```python
from build123d import *

# Parameters (mm, degrees)
F0_W     = 12.065
F0_H     = 4.572
F1_DEPTH = 17.272
F2_W     = 12.065
F2_H     = 2.794
F2_W_2   = 1.0795
F2_H_2   = 1.778
F3_DEPTH = 21.59


with BuildPart() as f1:
    # F0 (on Front) → F1 (new body)
    with BuildSketch(Plane.XZ):
        Rectangle(F0_W, F0_H)
    extrude(amount=F1_DEPTH)

    # F2 (on face) → F3 (join)
    with BuildSketch(Plane(origin=(0, 0, 0), x_dir=(-1, 0, 0), z_dir=(0, 1, 0))):
        with Locations((0, 0.889)):
            Rectangle(F2_W, F2_H)
        with Locations((6.57225, -1.397)):
            Rectangle(F2_W_2, F2_H_2)
        with Locations((0, -1.397)):
            Rectangle(F2_W, F2_H_2)
        with Locations((-6.57225, -1.397)):
            Rectangle(F2_W_2, F2_H_2)
    extrude(amount=F3_DEPTH)


solid = f1.part
```
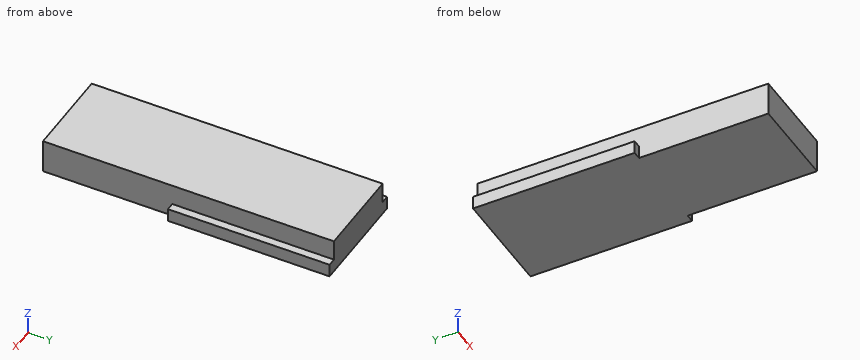
The model under review builds one solid part; all positions refer to its coordinate system, in mm. Round coordinates to 2 decimals unless told otherwise and drop trailing zeros. Order: outer loops, then holes, each group sorted by start corner. A loop starts at its lowest first (then second) coordinate and runs counter-clockwise, first axis right, second up. Notation, with made-up numbers: (77, 16) -> (103, 16) arc R27 cw to (103, 53) -> close; hole circle Ø11 at (0.5, 35). An arc over 180 degrees is marked (long way). Use a Markdown table: item, result.
Q1. Clearance check with flat-ended pins moving along their axes: P1, Ø1.5, axis at y = 0.5, z = 1.5, coming from the -X side; P2, Ø1.2, axis at x = 7, y = 8, coming from the +Z side. State where each tip first meets the part, or that it passes through.
Values:
| item | result |
|---|---|
| P1 | stops at x = -6.03 |
| P2 | stops at z = -0.51 |
Q2. We need section A-A on y = 12. Write out the cut boundary in (x, z).
Values:
| item | result |
|---|---|
| outline | (-7.11, -2.29) -> (7.11, -2.29) -> (7.11, -0.51) -> (6.03, -0.51) -> (6.03, 2.29) -> (-6.03, 2.29) -> (-6.03, -0.51) -> (-7.11, -0.51) -> close |
Q3. We need section C-C on z = 0.5. Write out the cut boundary in (x, y), then the cut area to 3 significant figures.
Values:
| item | result |
|---|---|
| outline | (-6.03, -17.27) -> (6.03, -17.27) -> (6.03, 21.59) -> (-6.03, 21.59) -> close |
| area | 469 mm^2 |
Q4. We need section B-B on z = -1.35. Write out the cut boundary in (x, y), then the cut area to 3 significant figures.
Values:
| item | result |
|---|---|
| outline | (-7.11, 0) -> (-6.03, 0) -> (-6.03, -17.27) -> (6.03, -17.27) -> (6.03, 0) -> (7.11, 0) -> (7.11, 21.59) -> (-7.11, 21.59) -> close |
| area | 515 mm^2 |
Q5. For line 1 (X direction, y = 8, z = 1), list the stretches that pass through material, from the lowest coordinate up.
Values:
| item | result |
|---|---|
| line 1 | x = -6.03 to 6.03 |
Q6. We need section D-D on y = -14. Write out the cut boundary in (x, z), then the cut area to 3 significant figures.
Values:
| item | result |
|---|---|
| outline | (-6.03, -2.29) -> (6.03, -2.29) -> (6.03, 2.29) -> (-6.03, 2.29) -> close |
| area | 55.2 mm^2 |
